The listing builds one solid part. Answer for the finished solid, in the listing's coordinates (mm). A direction names the side the tool comes from. Give positions to 0.01 mm unless a question says otherwise; leave off trailing zeros. Order: outer loops, then holes, each group sorted by start corner. A loop starts at its lowest first (then second) coordinate and runs counter-clockwise, first axis right, second up. Notation, with made-up numbers: (77, -15) -> (90, -15) arc R21 ccw to (90, -6) -> close; hole circle Ø3 at (26, 34). An arc over 180 degrees is marked (long way). Write item = value, one per line. Start each with the question number.
```python
from build123d import *

# Parameters (mm, degrees)
SKETCH1_R               = 15.5
BOSS_EXTRUDE1_DEPTH     = 62
CUT_EXTRUDE1_DEPTH      = 66.76093065
CUT_EXTRUDE1_DEPTH_BACK = 66.76093065


with BuildPart() as part:
    # Sketch1 → Boss-Extrude1 (new body)
    with BuildSketch(Plane.XY):
        Circle(SKETCH1_R)
    extrude(amount=BOSS_EXTRUDE1_DEPTH)

    # Sketch2 → Cut-Extrude1 (cut, two sides: drawn at the far end of the back side and taken through both)
    with BuildSketch(Plane(origin=(0, 0, 0), x_dir=(1, 0, 0), z_dir=(0, 1, 0)).offset(-CUT_EXTRUDE1_DEPTH_BACK)):
        Polygon((-15.5, -22.33712703), (-13.35, -24.5), (-13.35, -45.5), (-15.5, -47.66287297), align=None)
        Polygon((15.5, -47.66287297), (13.35, -45.5), (13.35, -24.5), (15.5, -22.33712703), align=None)
    extrude(amount=CUT_EXTRUDE1_DEPTH + CUT_EXTRUDE1_DEPTH_BACK, mode=Mode.SUBTRACT)


solid = part.part
```
Item 1: Flat-ended cylindrical pins translate along their axes: pin 1 (12.5 mm diameter, centred on y = 3.5, z = 33.5, fed in from +X); pin 2 (8 mm diameter, centred on y = -6.5, z = 15, fed in from -X); pin 3 (3 mm diameter, centred on x = 9, z = 27, fed in from -Y); pin 4 (1 mm diameter, centred on x = -0.5, z = 36.5, fed in from +Y). Find the tip coordinate at first contact, or state that the pin passes through.
Item 2: A cutting plane is placed at C-C, the plane x = 11.5. Write down the section's boundary in (y, z), plus the area to 3 significant figures.
Item 3: Consider L1, parallel to X at y = 4, z = 38; L2, parallel to X at y = -0.5, z = 54; L3, parallel to Y at x = -1.5, z = 57.5. Determine where each line is inside the solid, lowest interval first. Write a range as from..to.
Item 4: The mould has two halves that part along Z. Classify faces 1 (the flat face through (0, 0, 62)), 2 (the flat face through (-13.35, 0, 35)), 3 (the flat face through (0, 0, 0)), 4 (the flat face through (-14.171, -0.11, 46.326)): +Z half, -Z half, draft (parallel to the pull), parting line (faces both ways), or undercut.
Item 5: A cutting plane is placed at A-A, the plane y = 0. Write down the section's boundary in (x, z).
Item 6: A cutting plane is placed at D-D, the plane z = 48.5. Write down the section's boundary in (x, y), plus the area to 3 significant figures.
Item 7: Which of the six approach directions +Z, -Z, +X, -X, +Y, -Y give full straight-line access (tool end or side, diameter ignored) to faces 5 (the flat face through (-14.201, -0.11, 23.644)), 6 (the cylindrical face through (-11.4, 10.5, 30.6)), 7 (the flat face through (14.171, -0.11, 23.674))?
Item 8: A cutting plane is placed at B-B, the plane z = 34. Write down the section's boundary in (x, y), plus the area to 3 significant figures.
Check values:
q1.pin_1 = 13.35
q1.pin_2 = -15.3
q1.pin_3 = -13.56
q1.pin_4 = 15.5
q2.outline = (-10.39, 0) -> (10.39, 0) -> (10.39, 62) -> (-10.39, 62) -> close
q2.area = 1,290 mm^2
q3.L1 = -13.35..13.35
q3.L2 = -15.49..15.49
q3.L3 = -15.43..15.43
q4.face_1 = +Z half
q4.face_2 = undercut
q4.face_3 = -Z half
q4.face_4 = undercut
q5.outline = (-15.5, 0) -> (15.5, 0) -> (15.5, 22.34) -> (13.35, 24.5) -> (13.35, 45.5) -> (15.5, 47.66) -> (15.5, 62) -> (-15.5, 62) -> (-15.5, 47.66) -> (-13.35, 45.5) -> (-13.35, 24.5) -> (-15.5, 22.34) -> close
q6.outline = circle Ø31 at (0, 0)
q6.area = 755 mm^2
q7.face_5 = -X, +Y, -Y
q7.face_6 = +Z, -Z
q7.face_7 = +X, +Y, -Y
q8.outline = (-13.35, -7.88) arc R15.5 ccw to (13.35, -7.88) -> (13.35, 7.88) arc R15.5 ccw to (-13.35, 7.88) -> close
q8.area = 709 mm^2
